from build123d import *

# Parameters (mm, degrees)
SM_BASE_FLANGE_1_DEPTH = 198.3
FILLET_1_R             = 3
SKETCH_6_R             = 1.65
CUT_EXTRUDE_1_DEPTH    = 309.167389579
CUT_EXTRUDE_2_REACH    = 486.779
SKETCH_7_R             = 1.65
CHAMFER_2_SIZE         = 1.6


# Sheet-metal steps are written as plain solids
with BuildPart() as part:
    # Sketch 1 → Базовая кромка1 (new body)
    with BuildSketch(Plane.XY):
        with BuildLine():
            Line((-217.2, -66.1), (-217.2, 19.3))
            ThreePointArc((-217.2, 19.3), (-216.760660172, 20.360660172), (-215.7, 20.8))
            Line((-215.7, 20.8), (215.7, 20.8))
            ThreePointArc((215.7, 20.8), (216.760660172, 20.360660172), (217.2, 19.3))
            Line((217.2, 19.3), (217.2, -66.1))
            Line((217.2, -66.1), (218.7, -66.1))
            Line((218.7, -66.1), (218.7, 19.3))
            ThreePointArc((218.7, 19.3), (217.821320344, 21.421320344), (215.7, 22.3))
            Line((215.7, 22.3), (-215.7, 22.3))
            ThreePointArc((-215.7, 22.3), (-217.821320344, 21.421320344), (-218.7, 19.3))
            Line((-218.7, 19.3), (-218.7, -66.1))
            Line((-218.7, -66.1), (-217.2, -66.1))
        make_face()
    extrude(amount=SM_BASE_FLANGE_1_DEPTH)

    # Скругление1
    fillet_1_edges = [part.edges().sort_by_distance(p)[0] for p in [
        (-217.95, -66.1, 0),
        (217.95, -66.1, 0),
        (-217.95, -66.1, 198.3),
        (217.95, -66.1, 198.3),
    ]]
    fillet(fillet_1_edges, radius=FILLET_1_R)

    # Эскиз6 → Вырез-Вытянуть1 (cut, through all)
    with BuildSketch(Plane(origin=(0, 22.3, 0), x_dir=(1, 0, 0), z_dir=(0, 1, 0))):
        with Locations(Location((-150, -7, 0), (0, 0, 270))):
            Circle(SKETCH_6_R)
        with Locations(Location((150, -7, 0), (0, 0, 270))):
            Circle(SKETCH_6_R)
    cut_extrude_1 = extrude(amount=-CUT_EXTRUDE_1_DEPTH, mode=Mode.SUBTRACT)

    # Зеркальное отражение1: Вырез-Вытянуть1 across plane
    add(cut_extrude_1.mirror(Plane(origin=(0, 0, 99.15), x_dir=(1, 0, 0), z_dir=(0, 0, -1))), mode=Mode.SUBTRACT)

    # Вырез-Вытянуть2: up to this face of the body (flat: up to its plane)
    cut_extrude_2_end = Plane(part.part.faces().sort_by_distance((-218.7, -23.390410792, 99.15))[0])
    # Эскиз7 → Вырез-Вытянуть2 (cut, up to the picked face)
    with BuildSketch(Plane(origin=(218.7, 0, 0), x_dir=(0, 0, -1), z_dir=(1, 0, 0)), mode=Mode.PRIVATE) as cut_extrude_2_sk1:
        with Locations(Location((-154.15, -58.1, 0), (0, 0, 90))):
            Circle(SKETCH_7_R)
    cut_extrude_2_tool1 = split(extrude(cut_extrude_2_sk1.sketch, amount=-CUT_EXTRUDE_2_REACH, mode=Mode.PRIVATE), bisect_by=cut_extrude_2_end, keep=Keep.BOTH, mode=Mode.PRIVATE)
    # Эскиз7 → Вырез-Вытянуть2 (cut, up to the picked face)
    with BuildSketch(Plane(origin=(218.7, 0, 0), x_dir=(0, 0, -1), z_dir=(1, 0, 0)), mode=Mode.PRIVATE) as cut_extrude_2_sk2:
        with Locations(Location((-44.15, -58.1, 0), (0, 0, 90))):
            Circle(SKETCH_7_R)
    cut_extrude_2_tool2 = split(extrude(cut_extrude_2_sk2.sketch, amount=-CUT_EXTRUDE_2_REACH, mode=Mode.PRIVATE), bisect_by=cut_extrude_2_end, keep=Keep.BOTH, mode=Mode.PRIVATE)
    add(cut_extrude_2_tool1.solids().sort_by(Axis((218.7, -58.1, 154.15), (-1, 0, 0)))[0], mode=Mode.SUBTRACT)
    add(cut_extrude_2_tool2.solids().sort_by(Axis((218.7, -58.1, 44.15), (-1, 0, 0)))[0], mode=Mode.SUBTRACT)

    # Фаска2
    # the kernel refuses this chamfer: 1.6 mm, written as the material it takes off along each edge
    with BuildSketch(Plane(origin=(-218.7, -58.1, 44.15), x_dir=(0, 1, 0), z_dir=(0, 0, -1))) as chamfer_2_piece_1:
        Polygon((1.65 + CHAMFER_2_SIZE, 0), (1.65, CHAMFER_2_SIZE), (1.65, 0), align=None)
    revolve(axis=Axis((-218.7, -58.1, 44.15), (1, 0, 0)), mode=Mode.SUBTRACT)
    with BuildSketch(Plane(origin=(-218.7, -58.1, 154.15), x_dir=(0, 1, 0), z_dir=(0, 0, -1))) as chamfer_2_piece_2:
        Polygon((1.65 + CHAMFER_2_SIZE, 0), (1.65, CHAMFER_2_SIZE), (1.65, 0), align=None)
    revolve(axis=Axis((-218.7, -58.1, 154.15), (1, 0, 0)), mode=Mode.SUBTRACT)
    with BuildSketch(Plane(origin=(-150, 22.3, 191.3), x_dir=(0, 0, -1), z_dir=(-1, 0, 0))) as chamfer_2_piece_3:
        Polygon((1.65 + CHAMFER_2_SIZE, 0), (1.65, CHAMFER_2_SIZE), (1.65, 0), align=None)
    revolve(axis=Axis((-150, 22.3, 191.3), (0, -1, 0)), mode=Mode.SUBTRACT)
    with BuildSketch(Plane(origin=(-150, 22.3, 7), x_dir=(0, 0, 1), z_dir=(-1, 0, 0))) as chamfer_2_piece_4:
        Polygon((1.65 + CHAMFER_2_SIZE, 0), (1.65, -CHAMFER_2_SIZE), (1.65, 0), align=None)
    revolve(axis=Axis((-150, 22.3, 7), (0, 1, 0)), mode=Mode.SUBTRACT)
    with BuildSketch(Plane(origin=(150, 22.3, 7), x_dir=(0, 0, 1), z_dir=(-1, 0, 0))) as chamfer_2_piece_5:
        Polygon((1.65 + CHAMFER_2_SIZE, 0), (1.65, -CHAMFER_2_SIZE), (1.65, 0), align=None)
    revolve(axis=Axis((150, 22.3, 7), (0, 1, 0)), mode=Mode.SUBTRACT)
    with BuildSketch(Plane(origin=(218.7, -58.1, 44.15), x_dir=(0, 1, 0), z_dir=(0, 0, -1))) as chamfer_2_piece_6:
        Polygon((1.65 + CHAMFER_2_SIZE, 0), (1.65, -CHAMFER_2_SIZE), (1.65, 0), align=None)
    revolve(axis=Axis((218.7, -58.1, 44.15), (1, 0, 0)), mode=Mode.SUBTRACT)
    with BuildSketch(Plane(origin=(218.7, -58.1, 154.15), x_dir=(0, 1, 0), z_dir=(0, 0, -1))) as chamfer_2_piece_7:
        Polygon((1.65 + CHAMFER_2_SIZE, 0), (1.65, -CHAMFER_2_SIZE), (1.65, 0), align=None)
    revolve(axis=Axis((218.7, -58.1, 154.15), (1, 0, 0)), mode=Mode.SUBTRACT)
    with BuildSketch(Plane(origin=(150, 22.3, 191.3), x_dir=(0, 0, -1), z_dir=(-1, 0, 0))) as chamfer_2_piece_8:
        Polygon((1.65 + CHAMFER_2_SIZE, 0), (1.65, CHAMFER_2_SIZE), (1.65, 0), align=None)
    revolve(axis=Axis((150, 22.3, 191.3), (0, -1, 0)), mode=Mode.SUBTRACT)


solid = part.part
Source: CAD feature listing. Evaluate the final solid. Frame: model axes, mm. A direction names the side the tool comes from. Give positions to 0.01 mm unless a question says otherwise; leave off trailing zeros. Write each loop counter-clockwise with the first axis right and the second up, starting at its lowest first coordinate (ties: lowest second). Pieces come first, ordered by that corner, then holes. Notation, with made-up numbers: (-23.5, -35) - (27.5, -35) arc R29 cw to (27.5, 3) - close; hole circle Ø1 at (78.5, -1.75). An arc over 180 degrees is marked (long way). Write item = value, one per line. Start each with the question number.
Q1. Cut plane A-A, the plane y = 6.5. Return loops of the section in (x, z), then the cut area to 3 significant figures.
Q2. Cut plane C-C, the plane x = 133. Return loops of the section in (y, z).
Q3. Material intervals for probe 1 along X at (y, z) = (6.5, 135.5); probe 2 along Y at (x, z) = (7.5, 156.5); probe 3 along X at (y, z) = (-57, 42), sorted ascending.
Q4. Reachability of faces 4 (the flat face through (217.2, -23, 98)), 5 (the flat face through (-1, 21, 198.3)) from +Z, -Z, +X, -X, +Y, -Y: full face, straight path, thin tool, end or side. Return the list, or none.
Q5. Cut plane B-B, the plane z = 182.5. Return loops of the section in (x, y), then the cut area to 3 significant figures.
Q6. Draft query along X for faces 1 (the flat face through (218.7, -24, 98)), 2 (the flat face through (-1, 21, 0)), 3 (the flat face through (-217.2, -24, 98)). Return one class per face: +X half, -X half, draft (parallel to the pull), parting line (faces both ways), or undercut.
Computed values:
q1.outline = (-218.7, 0) - (-217.2, 0) - (-217.2, 198.3) - (-218.7, 198.3) - close; (217.2, 0) - (218.7, 0) - (218.7, 198.3) - (217.2, 198.3) - close
q1.area = 595 mm²
q2.outline = (20.8, 0) - (22.3, 0) - (22.3, 198.3) - (20.8, 198.3) - close
q3.probe_1 = -218.7 to -217.2, 217.2 to 218.7
q3.probe_2 = 20.8 to 22.3
q3.probe_3 = -217.87 to -217.2, 217.2 to 217.87
q4.face_4 = +Z, -Z, -Y
q4.face_5 = +Z, +X, -X, +Y, -Y
q5.outline = (-218.7, -66.1) - (-217.2, -66.1) - (-217.2, 19.3) arc R1.5 cw to (-215.7, 20.8) - (215.7, 20.8) arc R1.5 cw to (217.2, 19.3) - (217.2, -66.1) - (218.7, -66.1) - (218.7, 19.3) arc R3 ccw to (215.7, 22.3) - (-215.7, 22.3) arc R3 ccw to (-218.7, 19.3) - close
q5.area = 914 mm²
q6.face_1 = +X half
q6.face_2 = draft
q6.face_3 = undercut
